Input: part model. Units: mm. Frame: model coordinates. A direction names the side the tool comes from. Round coordinates to 2 decimals unless told otherwise and drop trailing zeros. Write each loop counter-clockwise with the first axis right and the second up, starting at its lowest first coordinate (ties: lowest second). Pieces come first, ordered by that corner, then holes. Notation, with made-up numbers: (-1.75, 71) -> (6.25, 71) arc R18 cw to (6.25, 104) -> close; hole circle Ø7 at (21.25, 18.5). An arc over 180 degrees is marked (long way). Use CSV: the item, a comma, the result in double quotes.
```python
from build123d import *

# Parameters (mm, degrees)
FILLET1_R            = 7.5
FILLET2_R            = 5
CUT_EXTRUDE4_DEPTH   = 40
CUT_EXTRUDE4_DRAFT   = -7
CUT_EXTRUDE4_2_DEPTH = 40
CUT_EXTRUDE4_2_DRAFT = -7
CUT_EXTRUDE4_3_DEPTH = 40
CUT_EXTRUDE4_3_DRAFT = -7
SKETCH4_R            = 4
CUT_EXTRUDE5_DEPTH   = 107.183802908


# Read off the part's stored shape, not the designer's step: Cut-Extrude4
with BuildPart() as part:
    # Sketch1 → Revolve1 (revolve)
    with BuildSketch(Plane(origin=(0, 0, 0), x_dir=(0, 0, -1), z_dir=(1, 0, 0)), mode=Mode.PRIVATE) as revolve1_sk:
        Polygon((0, 20), (-85, 20), (-85, 35), (-30, 35), (-30, 45), (-15, 45), (-15, 35), (0, 35), align=None)
    revolve(revolve1_sk.sketch.rotate(Axis((0, 0, 95.688392975), (0, 0, -1)), 90), axis=Axis((0, 0, 95.688392975), (0, 0, -1)))

    # Fillet1
    fillet1_edges = [part.edges().sort_by_distance(p)[0] for p in [
        (-35, 0, 15),
    ]]
    fillet(fillet1_edges, radius=FILLET1_R)

    # Fillet2
    fillet2_edges = [part.edges().sort_by_distance(p)[0] for p in [
        (-35, 0, 30),
    ]]
    fillet(fillet2_edges, radius=FILLET2_R)


with BuildPart() as cut_extrude4_tool:
    # Cut-Extrude4 outline → Cut-Extrude4 (with draft: the straight prism first)
    with BuildSketch(Plane.XY.offset(45)):
        with BuildLine():
            ThreePointArc((16.880866709, -30.660012054), (31.304951685, -15.652475842), (34.656529669, 4.891313865))
            ThreePointArc((34.656529669, 4.891313865), (27.252000961, -13.626000481), (16.880866709, -30.660012054))
        make_face()
    extrude(amount=CUT_EXTRUDE4_DEPTH)
    # Cut-Extrude4: the draft: its side faces are tilted about the plane it starts from
    cut_extrude4_sides = [cut_extrude4_tool.faces().sort_by_distance(p)[0] for p in [
        (27.252000961, -13.626000481, 65),
        (31.304951685, -15.652475842, 65),
    ]]
    draft(cut_extrude4_sides, Plane.XY.offset(45), CUT_EXTRUDE4_DRAFT)


with BuildPart() as part_1:
    add(part.part)

    # Cut-Extrude4: cut by cut_extrude4_tool
    add(cut_extrude4_tool.part, mode=Mode.SUBTRACT)


with BuildPart() as cut_extrude4_2_tool:
    # Cut-Extrude4 2 outline → Cut-Extrude4 2 (with draft: the straight prism first)
    with BuildSketch(Plane.XY.offset(45)):
        with BuildLine():
            ThreePointArc((-34.656529669, 4.891313865), (-31.304951685, -15.652475842), (-16.880866709, -30.660012054))
            ThreePointArc((-16.880866709, -30.660012054), (-27.252000961, -13.626000481), (-34.656529669, 4.891313865))
        make_face()
    extrude(amount=CUT_EXTRUDE4_2_DEPTH)
    # Cut-Extrude4 2: the draft: its side faces are tilted about the plane it starts from
    cut_extrude4_2_sides = [cut_extrude4_2_tool.faces().sort_by_distance(p)[0] for p in [
        (-31.304951685, -15.652475842, 65),
        (-27.252000961, -13.626000481, 65),
    ]]
    draft(cut_extrude4_2_sides, Plane.XY.offset(45), CUT_EXTRUDE4_2_DRAFT)


with BuildPart() as part_2:
    add(part_1.part)

    # Cut-Extrude4 2: cut by cut_extrude4_2_tool
    add(cut_extrude4_2_tool.part, mode=Mode.SUBTRACT)


with BuildPart() as cut_extrude4_3_tool:
    # Cut-Extrude4 3 outline → Cut-Extrude4 3 (with draft: the straight prism first)
    with BuildSketch(Plane.XY.offset(45)):
        with BuildLine():
            ThreePointArc((20.897837677, 28.076331321), (0, 35), (-20.897837677, 28.076331321))
            ThreePointArc((-20.897837677, 28.076331321), (0, 29.911382436), (20.897837677, 28.076331321))
        make_face()
    extrude(amount=CUT_EXTRUDE4_3_DEPTH)
    # Cut-Extrude4 3: the draft: its side faces are tilted about the plane it starts from
    cut_extrude4_3_sides = [cut_extrude4_3_tool.faces().sort_by_distance(p)[0] for p in [
        (0, 35, 65),
        (0, 29.911382436, 65),
    ]]
    draft(cut_extrude4_3_sides, Plane.XY.offset(45), CUT_EXTRUDE4_3_DRAFT)


with BuildPart() as part_3:
    add(part_2.part)

    # Cut-Extrude4 3: cut by cut_extrude4_3_tool
    add(cut_extrude4_3_tool.part, mode=Mode.SUBTRACT)

    # Sketch4 → Cut-Extrude5 (cut, through all)
    with BuildSketch(Plane.XY.offset(85)):
        with Locations((25.11473671, 14.5)):
            Circle(SKETCH4_R)
        with Locations((-25.11473671, 14.5)):
            Circle(SKETCH4_R)
        with Locations((0, -29)):
            Circle(SKETCH4_R)
    extrude(amount=-CUT_EXTRUDE5_DEPTH, mode=Mode.SUBTRACT)


solid = part_3.part
```
Item 1: Set-up query: faces 1 (the face through (33.1, -26.9, 15)), 2 (the face through (15, 15, 0)), 3 (the face through (29, -14, 45)), 4 (the face through (30.2, 26.5, 30)), 5 (the face through (-28, -14, 45)). Return all of +Z, -Z, +X, -X, +Y, -Y with unobstructed straight access to the full face (end or side cutting, diameter ignored); none if empty.
Worked answers:
face 1,"-Z"
face 2,"-Z, +X, -X, +Y, -Y"
face 3,"+Z, +X, -Y"
face 4,"+Z"
face 5,"+Z, -X, -Y"
Item 2: Section query D-D on z = 61. Return the cut outline in (x, y).
Worked answers:
outline,"(-33.81, 9.04) arc R117.95 ccw to (-13.05, -32.47) arc R35 ccw to (13.05, -32.47) arc R117.95 ccw to (33.81, 9.04) arc R35 ccw to (23.99, 25.48) arc R117.95 ccw to (-23.99, 25.48) arc R35 ccw to start; hole circle Ø8 at (-25.11, 14.5); hole circle Ø40 at (0, 0); hole circle Ø8 at (0, -29); hole circle Ø8 at (25.11, 14.5)"
Item 3: Section query A-A on x = 0. Return the cut outline in (y, z), plus the area to 3 significant figures.
Worked answers:
outline,"(-45, 15) -> (-42.5, 15) arc R7.5 cw to (-35, 7.5) -> (-35, 0) -> (-33, 0) -> (-33, 85) -> (-35, 85) -> (-35, 35) arc R5 cw to (-40, 30) -> (-45, 30) -> close; (-25, 0) -> (-20, 0) -> (-20, 85) -> (-25, 85) -> close; (20, 0) -> (35, 0) -> (35, 7.5) arc R7.5 cw to (42.5, 15) -> (45, 15) -> (45, 30) -> (40, 30) arc R5 cw to (35, 35) -> (35, 45) -> (29.91, 45) -> (25, 85) -> (20, 85) -> close"
area,"1,900 mm²"
Item 4: First-contact query: pin 1 Ø10.5 at (x, y) = (0, -29) entering from -Z; pin 2 Ø1.5 at (x, y) = (-28.5, -24) entering from +Z; pin 3 Ø12 at (x, z) = (-10, 55.5) entering from -Y; pin 4 Ø6.5 at (x, y) = (-25.11, 14.5) entering from +Z. Flat tips, straight axial feed; report the tip coordinate or a pass-through.
Worked answers:
pin 1,"stops at z = 0"
pin 2,"stops at z = 31.42"
pin 3,"stops at y = -34.77"
pin 4,"passes through"
Item 5: Section query B-B on z = 39. Return the cut outline in (x, y).
Worked answers:
outline,"circle Ø70 at (0, 0); hole circle Ø8 at (-25.11, 14.5); hole circle Ø40 at (0, 0); hole circle Ø8 at (0, -29); hole circle Ø8 at (25.11, 14.5)"
Item 6: Line query: line 1 (X direction, y = 1, z = 78); line 2 (X direction, y = 2.5, z = 37.5); line 3 (Y direction, x = 0, z = 52). Output: solid intervals per line, ascending.
Worked answers:
line 1,"x = -29.1 to -19.97, 19.97 to 29.1"
line 2,"x = -34.91 to -19.84, 19.84 to 34.91"
line 3,"y = -35 to -33, -25 to -20, 20 to 29.05"
Item 7: Section query C-C on z = 25. Return the cut outline in (x, y).
Worked answers:
outline,"circle Ø90 at (0, 0); hole circle Ø8 at (-25.11, 14.5); hole circle Ø40 at (0, 0); hole circle Ø8 at (0, -29); hole circle Ø8 at (25.11, 14.5)"
